from build123d import *

# Parameters (mm, degrees)
BOSS_EXTRUDE1_DEPTH      = 584.2
BOSS_EXTRUDE1_DEPTH_BACK = 1.27
CUT_EXTRUDE1_DEPTH       = 19.05
SKETCH3_W                = 585.47
SKETCH3_H                = 3.175
CUT_EXTRUDE2_DEPTH       = 2.54
SKETCH4_W                = 585.47
SKETCH4_H                = 3.175
CUT_EXTRUDE3_DEPTH       = 2.54
SKETCH5_W                = 585.47
SKETCH5_H                = 3.175
CUT_EXTRUDE4_DEPTH       = 2.54
SKETCH6_W                = 585.47
SKETCH6_H                = 3.175
CUT_EXTRUDE5_DEPTH       = 2.54
CUT_EXTRUDE6_DEPTH       = 591.801160784
CUT_EXTRUDE8_DEPTH       = 591.667532064
FILLET4_R                = 1.016
CUT_EXTRUDE9_DEPTH       = 591.667532064
FILLET5_R                = 1.016
SKETCH12_W               = 3.175
SKETCH12_H               = 508
CUT_EXTRUDE10_DEPTH      = 2.54
BOSS_EXTRUDE3_DEPTH      = 25.4
SKETCH13_W               = 5.588
SKETCH13_H               = 635
CUT_EXTRUDE11_DEPTH      = 5.08


with BuildPart() as part:
    # Sketch1 → Boss-Extrude1 (new, two sides: drawn at the far end of the back side and taken through both)
    with BuildSketch(Plane.XY.offset(-BOSS_EXTRUDE1_DEPTH_BACK)):
        Polygon((83.386650215, 0), (80.211650215, 0), (80.211650215, 0.254), (75.385650215, 0.254), (75.385650215, 0), (7.059650215, 0), (7.059650215, 0.254), (2.233650215, 0.254), (2.233650215, 0), (-0.941349785, 0), (-0.941349785, 25.4), (83.386650215, 25.4), align=None)
    extrude(amount=BOSS_EXTRUDE1_DEPTH + BOSS_EXTRUDE1_DEPTH_BACK)

    # Sketch2 → Cut-Extrude1 (cut)
    with BuildSketch(Plane.XZ):
        with BuildLine():
            Line((34.872650215, 27.305), (34.872650215, 555.625))
            ThreePointArc((34.872650215, 555.625), (41.222650215, 561.975), (47.572650215, 555.625))
            Line((47.572650215, 555.625), (47.572650215, 27.305))
            ThreePointArc((47.572650215, 27.305), (41.222650215, 20.955), (34.872650215, 27.305))
        make_face()
    extrude(amount=-CUT_EXTRUDE1_DEPTH, mode=Mode.SUBTRACT)

    # Sketch3 → Cut-Extrude2 (cut)
    with BuildSketch(Plane(origin=(83.386650215, 0, 0), x_dir=(0, 0, -1), z_dir=(1, 0, 0))):
        with Locations((-291.465, 20.6375)):
            Rectangle(SKETCH3_W, SKETCH3_H)
    extrude(amount=-CUT_EXTRUDE2_DEPTH, mode=Mode.SUBTRACT)

    # Sketch4 → Cut-Extrude3 (cut)
    with BuildSketch(Plane(origin=(83.386650215, 0, 0), x_dir=(0, 0, -1), z_dir=(1, 0, 0))):
        with Locations((-291.465, 4.7625)):
            Rectangle(SKETCH4_W, SKETCH4_H)
    extrude(amount=-CUT_EXTRUDE3_DEPTH, mode=Mode.SUBTRACT)

    # Sketch5 → Cut-Extrude4 (cut)
    with BuildSketch(Plane.ZY.offset(0.941349785)):
        with Locations((291.465, 4.7625)):
            Rectangle(SKETCH5_W, SKETCH5_H)
    extrude(amount=-CUT_EXTRUDE4_DEPTH, mode=Mode.SUBTRACT)

    # Sketch6 → Cut-Extrude5 (cut)
    with BuildSketch(Plane.ZY.offset(0.941349785)):
        with Locations((291.465, 20.6375)):
            Rectangle(SKETCH6_W, SKETCH6_H)
    extrude(amount=-CUT_EXTRUDE5_DEPTH, mode=Mode.SUBTRACT)

    # Sketch7 → Cut-Extrude6 (cut, through all)
    with BuildSketch(Plane(origin=(83.386650215, 0, 0), x_dir=(0, 0, -1), z_dir=(1, 0, 0))):
        with BuildLine():
            Line((-11.43, 9.5123), (-571.5, 9.5123))
            ThreePointArc((-571.5, 9.5123), (-574.6877, 12.7), (-571.5, 15.8877))
            Line((-571.5, 15.8877), (-11.43, 15.8877))
            ThreePointArc((-11.43, 15.8877), (-8.2423, 12.7), (-11.43, 9.5123))
        make_face()
    extrude(amount=-CUT_EXTRUDE6_DEPTH, mode=Mode.SUBTRACT)

    # Sketch10 → Cut-Extrude8 (cut, through all)
    with BuildSketch(Plane(origin=(0, 25.4, 0), x_dir=(1, 0, 0), z_dir=(0, 1, 0))):
        Polygon((41.222650215, -584.2), (47.572650215, -584.2), (47.572650215, -561.34), (34.872650215, -561.34), (34.872650215, -584.2), align=None)
    extrude(amount=-CUT_EXTRUDE8_DEPTH, mode=Mode.SUBTRACT)

    # Fillet4
    fillet4_edges = [part.edges().sort_by_distance(p)[0] for p in [
        (47.572650215, 20.64385, 561.34),
        (34.872650215, 20.64385, 561.34),
    ]]
    fillet(fillet4_edges, radius=FILLET4_R)

    # Sketch9 → Cut-Extrude9 (cut, through all)
    with BuildSketch(Plane.XZ):
        Polygon((47.572650215, -1.27), (34.872650215, -1.27), (34.872650215, 5.08), (41.222650215, 5.08), (47.572650215, 5.08), align=None)
    extrude(amount=-CUT_EXTRUDE9_DEPTH, mode=Mode.SUBTRACT)

    # Fillet5
    fillet5_edges = [part.edges().sort_by_distance(p)[0] for p in [
        (47.572650215, 12.7, 5.08),
        (34.872650215, 12.7, 5.08),
    ]]
    fillet(fillet5_edges, radius=FILLET5_R)

    # Sketch12 → Cut-Extrude10 (cut)
    with BuildSketch(Plane(origin=(0, 25.4, 0), x_dir=(1, 0, 0), z_dir=(0, 1, 0))):
        with Locations((33.505889839, -264.440775348)):
            Rectangle(SKETCH12_W, SKETCH12_H)
        Polygon((47.793389839, -10.440775348), (47.793389839, -13.508701224), (47.793389839, -20.346727485), (47.793389839, -518.440775348), (50.968389839, -518.440775348), (50.968389839, -10.440775348), align=None)
    extrude(amount=-CUT_EXTRUDE10_DEPTH, mode=Mode.SUBTRACT)

    # Sketch15 → Boss-Extrude3 (add)
    with BuildSketch(Plane.XY.offset(584.2)):
        Polygon((-0.941349785, 25.4), (34.872650215, 25.4), (34.872650215, 0), (7.059650215, 0), (7.059650215, 0.254), (2.233650215, 0.254), (2.233650215, 0), (-0.941349785, 0), (-0.941349785, 3.175), (1.598650215, 3.175), (1.598650215, 6.35), (-0.941349785, 6.35), (-0.941349785, 19.05), (1.598650215, 19.05), (1.598650215, 22.225), (-0.941349785, 22.225), align=None)
        Polygon((47.572650215, 0), (47.572650215, 25.4), (83.386650215, 25.4), (83.386650215, 22.225), (80.846650215, 22.225), (80.846650215, 19.05), (83.386650215, 19.05), (83.386650215, 6.35), (80.846650215, 6.35), (80.846650215, 3.175), (83.386650215, 3.175), (83.386650215, 0), (80.211650215, 0), (80.211650215, 0.254), (75.385650215, 0.254), (75.385650215, 0), align=None)
    extrude(amount=BOSS_EXTRUDE3_DEPTH)

    # Sketch13 → Cut-Extrude11 (cut)
    with BuildSketch(Plane(origin=(0, 25.4, 0), x_dir=(1, 0, 0), z_dir=(0, 1, 0))):
        with Locations((41.222650215, -302.540775348)):
            Rectangle(SKETCH13_W, SKETCH13_H)
    extrude(amount=-CUT_EXTRUDE11_DEPTH, mode=Mode.SUBTRACT)


solid = part.part
CAD build for the part. Positions are in the model's coordinates, mm. A direction names the side the tool comes from. Give positions to 0.01 mm unless a question says otherwise; leave off trailing zeros. Write each loop counter-clockwise with the first axis right and the second up, starting at its lowest first coordinate (ties: lowest second). Pieces come first, ordered by that corner, then holes. Notation, with made-up numbers: (-27, -28.75) -> (16, -28.75) arc R19 cw to (16, -22.75) -> close; hole circle Ø1 at (25.5, -28). An arc over 180 degrees is marked (long way). Return JSON: item names as keys, results as strings.
Item 1: Two-plate mould, pull along Y, no slides. Class faces 1 (the flat face through (51, 9.512, 288)), 2 (the flat face through (63, 25.4, 300)), 3 (the flat face through (66, 13, -1.27)): +Y half, -Y half, draft (parallel to the pull), parting line (faces both ways), or undercut.
Answer below:
{"face 1": "undercut", "face 2": "+Y half", "face 3": "draft"}
Item 2: Drop flat-ended pins along their axis: pin 1 (10 mm diameter, centred on y = 13, z = 429.5, fed in from +X); pin 2 (1 mm diameter, centred on y = 11.5, z = 84.5, fed in from -X); pin 3 (1.6 mm diameter, centred on y = 21, z = 214, fed in from +X); pin 4 (2 mm diameter, centred on y = 4.5, z = 457.5, fed in from -X). Give the stop position or say it passes through.
Answer below:
{"pin 1": "stops at x = 83.39", "pin 2": "passes through", "pin 3": "stops at x = 80.85", "pin 4": "stops at x = 1.6"}
Item 3: Tool access for faces 4 (the flat face through (41, 20, 561.34)), 5 (the flat face through (34.873, 5, 288)), 6 (the flat face through (18, 25.4, 300)), 7 (the flat face through (41, 13, 5.08)), 8 (the flat face through (51, 15.888, 295)): list every direction of +Z, -Z, +X, -X, +Y, -Y with a clear straight run to the whole face (end or side of a thin tool).
Answer below:
{"face 4": "+Z, +Y, -Y", "face 5": "-Y", "face 6": "+Z, -Z, +X, -X, +Y", "face 7": "-Z, +Y, -Y", "face 8": "+X, -X"}
Item 4: Drill centre lines: probe 1 along X at (y, z) = (23.75, 24); probe 2 along Y at (x, z) = (48.5, 104.5); probe 3 along Y at (x, z) = (72, 369). Where is each one in solid material? Low to high.
Answer below:
{"probe 1": "x = -0.94 to 31.92, 35.09 to 38.43, 44.02 to 47.79, 50.97 to 83.39", "probe 2": "y = 0 to 9.51, 15.89 to 22.86", "probe 3": "y = 0 to 9.51, 15.89 to 25.4"}
Item 5: Band-saw the part on B-B (z = 529). Give the number of separate pieces and of enclosed holes in the cut face, then the cut area to 3 significant figures.
Answer below:
{"separate pieces": "3", "enclosed holes": "0", "area": "1,380 mm2"}
Item 6: Band-saw the part on A-A (x = 20). List the corners of the cut face in (y, z), then the cut area to 3 significant figures.
Answer below:
{"outline": "(0, -1.27) -> (25.4, -1.27) -> (25.4, 609.6) -> (0, 609.6) -> close; hole (9.51, 11.43) arc R3.19 ccw to (15.89, 11.43) -> (15.89, 571.5) arc R3.19 ccw to (9.51, 571.5) -> close", "area": "11,900 mm2"}
